Source: CAD feature listing. Evaluate the final solid. Frame: model axes, mm. Face numbers are marked on the shaded views. A direction names the side the tool comes from. Coordinates: 2 decimals unless noted, no trailing zeros. Order: outer loops, then holes, each group sorted by start corner. A loop starts at its lowest first (then second) coordinate and runs counter-clockwise, first axis right, second up. Notation, with made-up numbers: (-15, 38.5) -> (4, 38.5) arc R12 cw to (4, 58.5) -> close; hole circle Ø4 at (42.5, -8.75). An arc over 180 degrees is marked (long way). Write item = value, one per line. Start each with the question number.
Item 1: Section query A-A (y = -1.45). Output: boundary loops of the cut face in (x, z).
Item 2: Set-up query: the marked faces 1 and 2. Return all of +Z, -Z, +X, -X, +Y, -Y with unobstructed straight access to the full face (end or side cutting, diameter ignored); none if empty.
Item 3: Section query B-B (x = -50). Output: boundary loops of the cut face in (y, z).
Item 4: Section query C-C (z = 27.5). Output: boundary loops of the cut face in (x, y).
Item 5: Section query D-D (x = -29.5). Output: boundary loops of the cut face in (y, z).
Item 6: Ray query, line 1 along Z through (x, y) = (-50, -1.9); line 2 along Z through (x, y) = (-40, -3.2); line 3 along X through (y, z) = (-0.75, 44.5). Return the intervals inside material, ascending. Write a range as [from, to].
Item 7: Contact query for flat-ended pins moving along their axis: pin 1 (1.5 mm diameter, centred on y = -2, z = 35.5, fed in from -X); pin 2 (1 mm diameter, centred on x = -59.5, y = -3.5, fed in from +Z). Output: stop coordinate, or through.
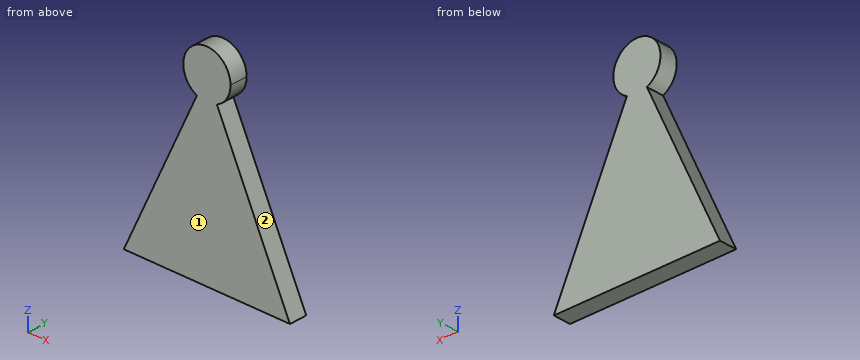
```python
from build123d import *

# Parameters (mm, degrees)
F1_DEPTH = 4.7


with BuildPart() as f1:
    # F0 (on Front) → F1 (new body)
    with BuildSketch(Plane.XZ):
        with BuildLine():
            Line((-47.77017605, 45.9924270552), (-67.3986524343, 3.9423387498))
            Line((-67.3986524343, 3.9423387498), (-22.7815322578, 3.9423387498))
            Line((-22.7815322578, 3.9423387498), (-42.4100088013, 45.9924270633))
            ThreePointArc((-42.4100088013, 45.9924270633), (-45.0900924247, 45.3977122077), (-47.77017605, 45.9924270552))
        make_face()
        with BuildLine():
            ThreePointArc((-38.753834, 51.7339706421), (-48.4935075231, 57.0785881851), (-47.77017605, 45.9924270552))
            Line((-47.77017605, 45.9924270552), (-45.0900924343, 51.7339706421))
            Line((-45.0900924343, 51.7339706421), (-42.4100088013, 45.9924270633))
            ThreePointArc((-42.4100088013, 45.9924270633), (-39.7454748862, 48.3305555615), (-38.753834, 51.7339706421))
        make_face()
        with BuildLine():
            Line((-45.0900924343, 51.7339706421), (-47.77017605, 45.9924270552))
            ThreePointArc((-47.77017605, 45.9924270552), (-45.0900924247, 45.3977122077), (-42.4100088013, 45.9924270633))
            Line((-42.4100088013, 45.9924270633), (-45.0900924343, 51.7339706421))
        make_face()
    extrude(amount=F1_DEPTH)


solid = f1.part
```
Computed:
q1.outline = (-67.4, 3.94) -> (-22.78, 3.94) -> (-42.41, 45.99) arc R6.34 ccw (long way) to (-47.77, 45.99) -> close
q2.face_1 = +Z, -Z, +X, -X, -Y
q2.face_2 = +X, +Y, -Y
q3.outline = (-4.7, 3.94) -> (0, 3.94) -> (0, 41.22) -> (-4.7, 41.22) -> close; (-4.7, 47.73) -> (0, 47.73) -> (0, 55.74) -> (-4.7, 55.74) -> close
q4.outline = (-56.4, -4.7) -> (-33.78, -4.7) -> (-33.78, 0) -> (-56.4, 0) -> close
q5.outline = (-4.7, 3.94) -> (0, 3.94) -> (0, 18.34) -> (-4.7, 18.34) -> close
q6.line_1 = [3.94, 41.22], [47.73, 55.74]
q6.line_2 = [3.94, 40.83], [47.96, 55.51]
q6.line_3 = [-48.47, -41.71]
q7.pin_1 = -53.02
q7.pin_2 = 21.93
